Source: CAD feature listing. Evaluate the final solid. Frame: model axes, mm. Face numbers are marked on the shaded views. A direction names the side the tool comes from. Give positions to 0.01 mm unless a question says otherwise; leave off trailing zeros. Write each loop counter-clockwise with the first axis right and the second up, starting at its lowest first coordinate (ties: lowest second). Pieces come first, ordered by that corner, then holes. Notation, with made-up numbers: (82, 4.25) -> (90, 4.25) arc R16 cw to (90, 33.25) -> close; hole circle Ø3 at (88.5, 64). An arc over 180 degrees is marked (long way). Write item = value, one per line.
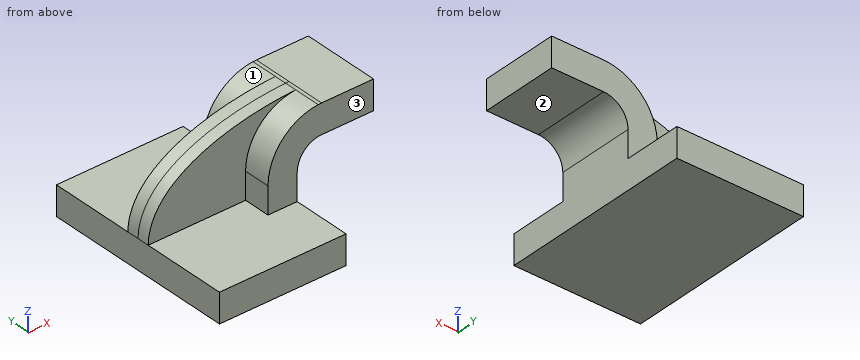
from build123d import *

# Parameters (mm, degrees)
F1_DEPTH = 63.5
F0_W     = 30.702464082
F0_H     = 19.05
F2_DEPTH = 25.4
F3_DEPTH = 7.9375


with BuildPart() as f1:
    # F0 (on Front) → F1 (new body, symmetric)
    with BuildSketch(Plane.XZ):
        Polygon((22.225, 9.525), (-41.275, 9.525), (-41.275, -9.525), (41.275, -9.525), (41.275, 9.525), align=None)
    extrude(amount=F1_DEPTH, both=True)

    # F0 (on Front) → F2 (join, symmetric)
    with BuildSketch(Plane.XZ):
        with BuildLine():
            Line((22.225, 27.0002), (22.225, 9.525))
            Line((22.225, 9.525), (41.275, 9.525))
            Line((41.275, 9.525), (41.275, 27.0002))
            ThreePointArc((41.275, 27.0002), (45.9246798487, 38.2255201513), (57.15, 42.8752))
            Line((57.15, 42.8752), (60.325, 42.8752))
            Line((60.325, 42.8752), (60.325, 61.9252))
            Line((60.325, 61.9252), (57.15, 61.9252))
            add(Edge.make_bspline(
                [(54.9349397203, 61.8548859541), (55.6723551603, 61.8816525899), (56.410751637, 61.905089585), (57.15, 61.9252)],
                knots=[109.884057266, 109.884057266, 109.884057266, 109.884057266, 111.5045361635, 111.5045361635, 111.5045361635, 111.5045361635], degree=3))
            ThreePointArc((54.9349397203, 61.8548859541), (31.6831921389, 50.899934776), (22.225, 27.0002))
        make_face()
        with Locations((75.676232041, 52.4002)):
            Rectangle(F0_W, F0_H)
    extrude(amount=F2_DEPTH, both=True)

    # F0 (on Front) → F3 (join, symmetric)
    with BuildSketch(Plane.XZ):
        with BuildLine():
            add(Edge.make_bspline(
                [(-41.275, 9.525), (-40.5618331855, 42.9146462333), (4.9310793981, 60.0398505673), (54.9349397203, 61.8548859541)],
                knots=[0, 0, 0, 0, 109.884057266, 109.884057266, 109.884057266, 109.884057266], degree=3))
            Line((-41.275, 9.525), (22.225, 9.525))
            Line((22.225, 9.525), (22.225, 27.0002))
            ThreePointArc((22.225, 27.0002), (31.6831921389, 50.899934776), (54.9349397203, 61.8548859541))
        make_face()
    extrude(amount=F3_DEPTH, both=True)


solid = f1.part
(1) First-contact query: pin 1 (1 mm diameter, centred on x = 12.5, y = -50.5, fed in from +Z) (3 decimals); pin 2 (8 mm diameter, centred on x = 44.5, z = 28, fed in from -Y); pin 3 (5 mm diameter, centred on y = 14.5, z = 19, fed in from -X) (3 decimals). Flat tips, straight axial feed; report the tip coordinate or a pass-through.
Values follow:
pin_1 = 9.525
pin_2 = -25.4
pin_3 = 22.225
(2) Section query B-B (z = 6). Return loops of the section in (x, y) (3 decimals), plus the area to 3 significant figures.
Values follow:
outline = (-41.275, -63.5) -> (41.275, -63.5) -> (41.275, 63.5) -> (-41.275, 63.5) -> close
area = 10,500 mm2
(3) Material intervals for line 1 (Z direction, x = -13.5, y = -44) (3 decimals); line 2 (X direction, y = 53, z = -4.5) (3 decimals); line 3 (Y direction, x = 45, z = 44), sorted ascending.
Values follow:
line_1 = -9.525 to 9.525
line_2 = -41.275 to 41.275
line_3 = -25.4 to 25.4
(4) Access query for the marked faces 1, 2 and 3. Directions: +Z, -Z, +X, -X, +Y, -Y. A direction counts if a zero-diameter tool reaches every point of the face in a straight line with its end or side. Return the directions, or none.
Values follow:
face_1 = +Z, -X, +Y
face_2 = -Z, +X, +Y, -Y
face_3 = +Z, +X, -X, -Y
(5) Section query A-A (x = 75). Return loops of the section in (y, z), plus the area to 3 significant figures.
Values follow:
outline = (-25.4, 42.88) -> (25.4, 42.88) -> (25.4, 61.93) -> (-25.4, 61.93) -> close
area = 968 mm2
